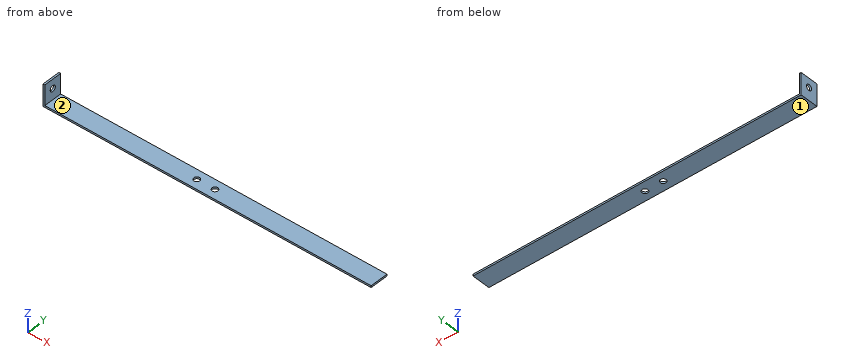
Autodesk Inventor part; units mm, degrees
ref_plane "YZ Plane" through (0, 0, 0) normal (1, 0, 0) x (0, 1, 0)
ref_plane "XZ Plane" through (0, 0, 0) normal (0, 1, 0) x (-1, 0, 0)
ref_plane "XY Plane" through (0, 0, 0) normal (0, 0, 1) x (1, 0, 0)
sketch "スケッチ1" plane through (0, 0, 0) normal (0, 0, 1) x (1, 0, 0)
  line L0 (-17.6, 4.0667) -> (162.4, 4.0667)
  line L1 (162.4, 4.0667) -> (162.4, -5.9333)
  line L2 (162.4, -5.9333) -> (-17.6, -5.9333)
  line L3 (-17.6, -5.9333) -> (-17.6, 4.0667)
  point P0 (0, 0)
  dimension "d0" = 10
  dimension "d1" = 180
extrude "押し出し1" add sketch "スケッチ1" along normal blind 1
sketch "スケッチ3" plane through (0, 0, 1) normal (0, 0, 1) x (1, 0, 0)
  circle A0 centre (62.4, -0.9333) radius 1.5
  line L0 (-17.6, 4.0667) -> (-17.6, -5.9333)
  line L1 (-17.6, -5.9333) -> (162.4, -5.9333)
  line L2 (162.4, 4.0667) -> (-17.6, 4.0667)
  point P0 (0, 0)
  point P1 (72.4, -0.9333)
  dimension "d14" = 3
  dimension "d15" = 80
  dimension "d16" = 5
  dimension "d24" = 10
  dimension "d25" = 5
hole "穴2" at (62.4, -0.9333, 1) at (72.4, -0.9333, 1) direction (0, 0, -1) diameter 3.2 end through all
sketch "スケッチ4" plane through (0, 0, 1) normal (0, 0, 1) x (1, 0, 0)
  line L0 (-17.6, -5.9333) -> (162.4, -5.9333)
  line L1 (-17.6, 4.0667) -> (-16.6, 4.0667)
  line L2 (-16.6, 4.0667) -> (-16.6, -5.9333)
  line L3 (-16.6, -5.9333) -> (-17.6, -5.9333)
  line L4 (-17.6, -5.9333) -> (-17.6, 4.0667)
  point P0 (0, 0)
  dimension "d26" = 1
extrude "押し出し2" add sketch "スケッチ4" along normal blind 11
sketch "スケッチ5" plane through (-16.6, -5.9333, 1) normal (1, 0, 0) x (0, 0, -1)
  line L0 (-11, 0) -> (-11, 10)
  line L1 (0, 0) -> (-11, 0)
  point P0 (1, 5.9333)
  point P1 (-6, 5)
  dimension "d29" = 5
  dimension "d30" = 5
hole "穴3" at (-16.6, -0.9333, 7) direction (-1, 0, 0) diameter 3.2 end through all
properties part number "爪２" material "アルミニウム 6061"
CAD build for the part. Positions are in the model's coordinates, mm. Face numbers are marked on the shaded views. A direction names the side the tool comes from. Coordinates: 2 decimals unless noted, no trailing zeros. Order: outer loops, then holes, each group sorted by start corner. A loop starts at its lowest first (then second) coordinate and runs counter-clockwise, first axis right, second up.
Item 1: Drill centre lines: L1, parallel to Y at x = 62.4, z = 0.85; L2, parallel to Z at x = 7, y = 3.5; L3, parallel to X at y = 1, z = 7.75. Where is each one in solid material? Low to high.
Check sheet entries:
L1: y = -5.93 to -2.53, 0.67 to 4.07
L2: z = 0 to 1
L3: x = -17.6 to -16.6
Item 2: 3-axis set-ups, long thin cutter, end or side, ignore diameter. For the marked faces 1 and 2: which of +Z, -Z, +X, -X, +Y, -Y reach the whole face in a straight line?
Check sheet entries:
face 1: -Z, +X, -X, +Y, -Y
face 2: +Z, +X, +Y, -Y
Item 3: Band-saw the part on A-A on z = 7. List the corners of the cut face in (x, y).
Check sheet entries:
outline: (-17.6, -5.93) - (-16.6, -5.93) - (-16.6, -2.53) - (-17.6, -2.53) - close; (-17.6, 0.67) - (-16.6, 0.67) - (-16.6, 4.07) - (-17.6, 4.07) - close
Item 4: Band-saw the part on B-B on x = 72.4. List the corners of the cut face in (y, z).
Check sheet entries:
outline: (-5.93, 0) - (-2.53, 0) - (-2.53, 1) - (-5.93, 1) - close; (0.67, 0) - (4.07, 0) - (4.07, 1) - (0.67, 1) - close
Item 5: Pin check, flat tips, straight feed: pin 1 Ø1.5 at (y, z) = (1, 10) entering from +X; pin 2 Ø4 at (x, y) = (62.4, -0.93) entering from +Z. Stop position of each tip, or through.
Check sheet entries:
pin 1: stops at x = -16.6
pin 2: stops at z = 1
Item 6: Band-saw the part on C-C on y = -4. List the corners of the cut face in (x, z), plus the area to 3 significant figures.
Check sheet entries:
outline: (-17.6, 0) - (162.4, 0) - (162.4, 1) - (-16.6, 1) - (-16.6, 12) - (-17.6, 12) - close
area: 191 mm2
